```python
from build123d import *

# Parameters (mm, degrees)
CHANFREIN1_SIZE = 0.5


with BuildPart() as part:
    # Esquisse1 → Base-Révolution (revolve)
    with BuildSketch(Plane.XY, mode=Mode.PRIVATE) as base_r_volution_sk:
        with BuildLine():
            Line((0, 0), (0, 3))
            Line((0, 3), (19, 3))
            Line((19, 3), (25, 2))
            Line((25, 2), (25, 3))
            Line((25, 3), (26.645751311, 3))
            ThreePointArc((26.645751311, 3), (27.645751311, 1.645751311), (28, 0))
            Line((28, 0), (0, 0))
        make_face()
    revolve(base_r_volution_sk.sketch.rotate(Axis((0, 0, 0), (1, 0, 0)), 90), axis=Axis((0, 0, 0), (1, 0, 0)))

    # Chanfrein1
    chanfrein1_edges = [part.edges().sort_by_distance(p)[0] for p in [
        (0, 0, -3),
    ]]
    chamfer(chanfrein1_edges, length=CHANFREIN1_SIZE)


solid = part.part
```
For this review, take the finished solid that the model builds, in its own axes (mm). A direction names the side the tool comes from. Give positions to 0.01 mm unless a question says otherwise; leave off trailing zeros. Write each loop counter-clockwise with the first axis right and the second up, starting at its lowest first coordinate (ties: lowest second). Pieces come first, ordered by that corner, then holes. Notation, with made-up numbers: M 32,89 L 41,89 A18 ccw 41,107 Z; hole C -6.75,-24 d9. An arc over 180 degrees is marked long. One line per item, written item: value.
1) For P1, Ø2, axis at x = 21.5, z = 1, coming from the -Y side; P2, Ø1.5, axis at y = -2.5, z = 2.5, coming from the -X side; P3, Ø2, axis at x = 10.5, y = 2, coming from the +Z side, all flat-tipped, find the tip position at first contact; note any pin that passes through.
Results are:
P1: stops at y = -2.69
P2: stops at x = 0.29
P3: stops at z = 2.83
2) The part is to be moulded in two halves that separate along X. For faces 3 (the cylindrical face through (9.88, -0.9, 2.86)), 4 (the flat face through (0, 0, 0)), 5 (the conical face through (22.71, -2.01, 1.28)), say which applies: +X half, -X half, draft (parallel to the pull), parting line (faces both ways), or undercut.
Results are:
face 3: draft
face 4: -X half
face 5: undercut
3) Take a section at D-D, the plane x = 5.5. Write out the cut boundary in (y, z).
Results are:
outline: C 0,0 d6
4) For faces 1 (the cylindrical face through (25.83, -0.9, 2.86)), 2 (the flat face through (25, 2, -1)), list the 3-axis set-ups (+Z, -Z, +X, -X, +Y, -Y) from which the entire face can be reached by the end or side of a thin tool; tool diameter is ignored.
Results are:
face 1: +X, -X
face 2: none
5) For line 1 (Z direction, x = 21, y = -1.5); line 2 (X direction, y = 1.5, z = 1); line 3 (X direction, y = 1.25, z = 0), list the stretches that pass through material, from the lowest coordinate up. Write a range as from..to.
Results are:
line 1: z = -2.2..2.2
line 2: x = 0..27.57
line 3: x = 0..27.8
6) Take a section at C-C, the plane x = 22. Write out the cut boundary in (y, z), then the cut area to 3 significant figures.
Results are:
outline: C 0,0 d5
area: 19.6 mm²
7) Take a section at A-A, the plane y = 0. Write out the cut boundary in (x, z), then the cut area to 3 significant figures.
Results are:
outline: M 0,-2.5 L 0.5,-3 L 19,-3 L 25,-2 L 25,-3 L 26.65,-3 A4 ccw 26.65,3 L 25,3 L 25,2 L 19,3 L 0.5,3 L 0,2.5 Z
area: 159 mm²
